Can you work these out from the model? Positions are in its coordinate system, mm. Face numbers are marked on the shaded views. A direction names the side the tool comes from. Round coordinates to 2 decimals unless told otherwise and drop trailing zeros. Loops run counter-clockwise (first coordinate to the right, second up) from the corner with the lowest first, then second, coordinate; pieces in that order, holes last.
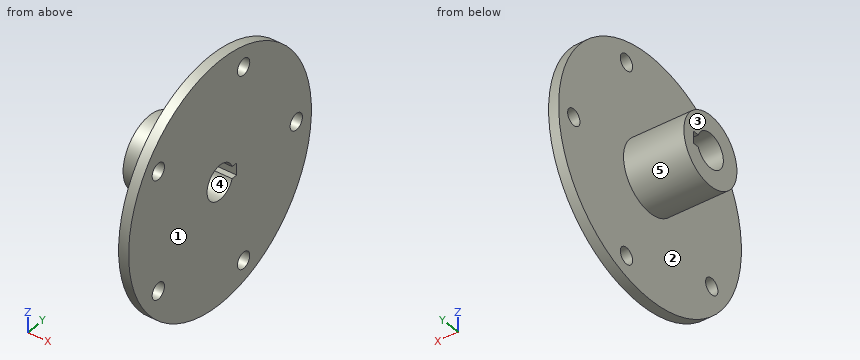
```python
from build123d import *

# Parameters (mm, degrees)
SKETCH1_R           = 60.325
BOSS_EXTRUDE1_DEPTH = 5
SKETCH2_R           = 4.064
CUT_EXTRUDE1_DEPTH  = 86.458827806
SKETCH11_R          = 17.5
BOSS_EXTRUDE3_DEPTH = 30
CUT_EXTRUDE5_DEPTH  = 93.212858377


with BuildPart() as part:
    # Sketch1 → Boss-Extrude1 (new body)
    with BuildSketch(Plane(origin=(0, 0, 0), x_dir=(0, 0, -1), z_dir=(1, 0, 0))):
        Circle(SKETCH1_R)
    extrude(amount=-BOSS_EXTRUDE1_DEPTH)

    # Sketch2 → Cut-Extrude1 (cut, through all)
    with BuildSketch(Plane(origin=(0, 0, 0), x_dir=(0, 0, -1), z_dir=(1, 0, 0))):
        with Locations((0, 50.342959834)):
            Circle(SKETCH2_R)
        with Locations((47.879, 15.556830136)):
            Circle(SKETCH2_R)
        with Locations((29.590849347, -40.728310053)):
            Circle(SKETCH2_R)
        with Locations((-29.590849347, -40.728310053)):
            Circle(SKETCH2_R)
        with Locations((-47.879, 15.556830136)):
            Circle(SKETCH2_R)
    extrude(amount=-CUT_EXTRUDE1_DEPTH, mode=Mode.SUBTRACT)

    # Sketch11 → Boss-Extrude3 (add)
    with BuildSketch(Plane.ZY.offset(5)):
        with Locations(Location((0, 0, 0), (0, 0, 180))):
            Circle(SKETCH11_R)
    extrude(amount=BOSS_EXTRUDE3_DEPTH)

    # Sketch12 → Cut-Extrude5 (cut, through all)
    with BuildSketch(Plane.ZY.offset(35)):
        with BuildLine():
            Line((0, 11.006403687), (-3, 11.006403687))
            Line((-3, 11.006403687), (-3, 8.006403687))
            ThreePointArc((-3, 8.006403687), (0, -8.55), (3, 8.006403687))
            Line((3, 8.006403687), (3, 11.006403687))
            Line((3, 11.006403687), (0, 11.006403687))
        make_face()
    extrude(amount=-CUT_EXTRUDE5_DEPTH, mode=Mode.SUBTRACT)


solid = part.part
```
(1) Suppose I cut it at D-D (x = -12.5). Write out the boundary of the cut face in (y, z).
(2) Suppose I cut it at C-C (y = -38.5). Write out the boundary of the cut face in (x, z).
(3) Suppose I cut it at A-A (z = 0). Write out the boundary of the cut face in (x, y) (3 decimals), then the cut area to 3 significant figures.
(4) Which directions (+Z, -Z, +X, -X, +Y, -Y) give clear straight access to the entire face, cutting with the end or side of a thin tool? Please do the marked faces 1 and 2.
(5) If I drill on line 1 (Z direction, x = -15, y = -0.5); line 2 (X direction, y = -34, z = -16.5); line 3 (Z direction, x = -32.5, y = -5), over which ranges is the centre line in solid material (lowest first)?
(6) For pin 1 (0.9 mm diameter, centred on x = -14, y = 10, fed in from +Z); pin 2 (3.5 mm diameter, centred on x = -14.5, y = 9.5, fed in from -Z); pin 3 (6 mm diameter, centred on y = -31, z = -35, fed in from -X), each with a flat end and sliding along its axis, tell me the tip position at first contact or that it passes through.
(7) Suppose I cut it at B-B (y = 0). Write out the boundary of the cut face in (x, z) (3 decimals).
(8) We'd pull the mould along Y, two halves only. Please class the marked faces 3, 4 and 5: released by +Y, released by -Y, zero draft, split by the parting line, or undercut.
Check result:
1. outline: circle Ø35 at (0, 0); hole (8.01, -3) - (11.01, -3) - (11.01, 3) - (8.01, 3) arc R8.55 ccw (long way) to start
2. outline: (-5, -46.44) - (0, -46.44) - (0, -32.99) - (-5, -32.99) - close; (-5, -26.19) - (0, -26.19) - (0, 26.19) - (-5, 26.19) - close; (-5, 32.99) - (0, 32.99) - (0, 46.44) - (-5, 46.44) - close
3. outline: (-35, -17.5) - (-5, -17.5) - (-5, -60.325) - (0, -60.325) - (0, -8.55) - (-35, -8.55) - close; (-35, 11.006) - (0, 11.006) - (0, 46.279) - (-5, 46.279) - (-5, 17.5) - (-35, 17.5) - close; (-5, 54.407) - (0, 54.407) - (0, 60.325) - (-5, 60.325) - close
3. area: 928 mm2
4. face 1: +Z, -Z, +X, +Y, -Y
4. face 2: -X
5. line 1: z = -17.49 to -8.54, 8.54 to 17.49
5. line 2: x = -5 to 0
5. line 3: z = -16.77 to -6.94, 6.94 to 16.77
6. pin 1: stops at z = 14.66
6. pin 2: stops at z = -15.69
6. pin 3: stops at x = -5
7. outline: (-35, -17.5) - (-5, -17.5) - (-5, -60.325) - (0, -60.325) - (0, -8.55) - (-35, -8.55) - close; (-35, 8.55) - (0, 8.55) - (0, 60.325) - (-5, 60.325) - (-5, 17.5) - (-35, 17.5) - close
8. face 3: zero draft
8. face 4: undercut
8. face 5: split by the parting line
